from build123d import *

# Parameters (mm, degrees)
F0_W     = 66.675
F0_H     = 53.18125
F1_DEPTH = 2.54
F3_DEPTH = 25.4
F4_R     = 1.5875
F5_DEPTH = 25.4


with BuildPart() as f1:
    # F0 (on Front) → F1 (new body)
    with BuildSketch(Plane.XZ):
        Rectangle(F0_W, F0_H)
    extrude(amount=F1_DEPTH)

    # F2 (on face) → F3 (cut)
    with BuildSketch(Plane.XZ.offset(2.54)):
        Polygon((33.3375, 26.590625), (27.78125, 26.590625), (30.559375, 23.8125), (30.559375, 13.890625), (33.3375, 11.1125), align=None)
        Polygon((33.3375, -26.590625), (33.3375, -21.828125), (30.559375, -24.60625), (30.559375, -26.590625), align=None)
    extrude(amount=-F3_DEPTH, mode=Mode.SUBTRACT)

    # F4 (on face) → F5 (cut)
    with BuildSketch(Plane.XZ.offset(2.54)):
        with Locations((30.95625, 8.331274)):
            Circle(F4_R)
        with Locations((30.559375, -17.065625)):
            Circle(F4_R)
        with Locations((-18.25625, -23.8125)):
            Circle(F4_R)
        with Locations((-18.25625, 23.8125)):
            Circle(F4_R)
    extrude(amount=-F5_DEPTH, mode=Mode.SUBTRACT)


solid = f1.part
Build history of the part. All positions in model axes, mm. A direction names the side the tool comes from. Round coordinates to 2 decimals unless told otherwise and drop trailing zeros. Loops run counter-clockwise (first coordinate to the right, second up) from the corner with the lowest first, then second, coordinate; pieces in that order, holes last. Notation, with made-up numbers: (42.5, 11) -> (83.5, 11) arc R13 cw to (83.5, 19) -> close; hole circle Ø9 at (-2, 81). An arc over 180 degrees is marked (long way). Answer in a Markdown table with one row per item.
Item 1: Saw through at A-A (x = -19). Write the cut outline in (y, z) (3 decimals), and give its area (3 significant figures).
Answers below:
| item | result |
|---|---|
| outline | (-2.54, -26.591) -> (0, -26.591) -> (0, -25.215) -> (-2.54, -25.215) -> close; (-2.54, -22.41) -> (0, -22.41) -> (0, 22.41) -> (-2.54, 22.41) -> close; (-2.54, 25.215) -> (0, 25.215) -> (0, 26.591) -> (-2.54, 26.591) -> close |
| area | 121 mm² |
Item 2: Which spindle directions (+Z, -Z, +X, -X, +Y, -Y) get a long thin tool onto all of the face, cutting with end or side? Do faces 1 (the cylindrical face through (-17.52, -1.29, -25.22)), 2 (the flat face through (30.559, -1, -26)). Say none if no direction does.
Answers below:
| item | result |
|---|---|
| face 1 | +Y, -Y |
| face 2 | -Z, +X, +Y, -Y |
Item 3: Pin check, flat tip, straight feed: pin 1 (0.6 mm diameter, centred on y = -1.5, z = -25, fed in from +X). Stop position of the tip, or through.
Answers below:
| item | result |
|---|---|
| pin 1 | stops at x = 30.56 |
Item 4: Mould opens along X. For faces 3 (the cylindrical face through (32.42, -1.29, 7.72)), 4 (the flat face through (30.559, -1, 19)), 5 (the flat face through (0, -2.54, 0)), 6 (the cylindrical face through (-17.524, -1.288, 22.404)) say: +X half, -X half, draft (parallel to the pull), parting line (faces both ways), or undercut.
Answers below:
| item | result |
|---|---|
| face 3 | undercut |
| face 4 | +X half |
| face 5 | draft |
| face 6 | undercut |
Item 5: Saw through at C-C (z = 16.5). Write the cut outline in (x, y), and give its area (3 significant figures).
Answers below:
| item | result |
|---|---|
| outline | (-33.34, -2.54) -> (30.56, -2.54) -> (30.56, 0) -> (-33.34, 0) -> close |
| area | 162 mm² |
Item 6: Saw through at B-B (y = -1.9). Write the cut outline in (x, z) (1 decimal).
Answers below:
| item | result |
|---|---|
| outline | (-33.3, -26.6) -> (30.6, -26.6) -> (30.6, -24.6) -> (33.3, -21.8) -> (33.3, 11.1) -> (30.6, 13.9) -> (30.6, 23.8) -> (27.8, 26.6) -> (-33.3, 26.6) -> close; hole circle Ø3.2 at (-18.3, -23.8); hole circle Ø3.2 at (-18.3, 23.8); hole circle Ø3.2 at (30.6, -17.1); hole circle Ø3.2 at (31, 8.3) |
Item 7: Drill centre lines: L1, parallel to Z at x = 30.5, y = -1.65; L2, parallel to X at y = -0.6, z = 18; L3, parallel to X at y = -2, z = 9. Where is each one in solid material? Low to high. Write a range as [from, to].
Answers below:
| item | result |
|---|---|
| L1 | z = [-26.59, -18.65], [-15.48, 6.81], [9.85, 23.87] |
| L2 | x = [-33.34, 30.56] |
| L3 | x = [-33.34, 29.52], [32.4, 33.34] |
